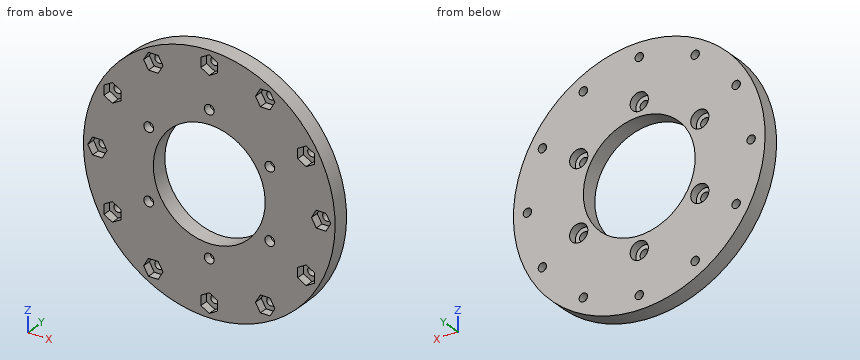
```python
from build123d import *

# Parameters (mm, degrees)
SKETCH1_R           = 45
BOSS_EXTRUDE1_DEPTH = 6
SKETCH3_R           = 1.75
CUT_EXTRUDE1_DEPTH  = 64.921827258
SKETCH4_R           = 3.25
CUT_EXTRUDE2_DEPTH  = 3
SKETCH5_R           = 1.5
CUT_EXTRUDE3_DEPTH  = 64.921827258
CUT_EXTRUDE4_DEPTH  = 3
SKETCH9_R           = 20
CUT_EXTRUDE5_DEPTH  = 64.921827258


with BuildPart() as part:
    # Sketch1 → Boss-Extrude1 (new body)
    with BuildSketch(Plane(origin=(0, 0, 0), x_dir=(1, 0, 0), z_dir=(0, 1, 0))):
        with Locations(Location((0, 0, 0), (0, 0, 270))):
            Circle(SKETCH1_R)
    extrude(amount=BOSS_EXTRUDE1_DEPTH)

    # Sketch3 → Cut-Extrude1 (cut, through all)
    with BuildSketch(Plane(origin=(0, 6, 0), x_dir=(1, 0, 0), z_dir=(0, 1, 0))):
        with Locations(Location((0, -25, 0), (0, 0, 270))):
            Circle(SKETCH3_R)
        with Locations(Location((-21.650635095, -12.5, 0), (0, 0, 270))):
            Circle(SKETCH3_R)
        with Locations(Location((-21.650635095, 12.5, 0), (0, 0, 270))):
            Circle(SKETCH3_R)
        with Locations(Location((0, 25, 0), (0, 0, 270))):
            Circle(SKETCH3_R)
        with Locations(Location((21.650635095, 12.5, 0), (0, 0, 270))):
            Circle(SKETCH3_R)
        with Locations(Location((21.650635095, -12.5, 0), (0, 0, 270))):
            Circle(SKETCH3_R)
    extrude(amount=-CUT_EXTRUDE1_DEPTH, mode=Mode.SUBTRACT)

    # Sketch4 → Cut-Extrude2 (cut)
    with BuildSketch(Plane(origin=(0, 6, 0), x_dir=(1, 0, 0), z_dir=(0, 1, 0))):
        with Locations(Location((0, -25, 0), (0, 0, 270))):
            Circle(SKETCH4_R)
        with Locations(Location((-21.650635095, -12.5, 0), (0, 0, 270))):
            Circle(SKETCH4_R)
        with Locations(Location((-21.650635095, 12.5, 0), (0, 0, 270))):
            Circle(SKETCH4_R)
        with Locations(Location((0, 25, 0), (0, 0, 270))):
            Circle(SKETCH4_R)
        with Locations(Location((21.650635095, 12.5, 0), (0, 0, 270))):
            Circle(SKETCH4_R)
        with Locations(Location((21.650635095, -12.5, 0), (0, 0, 270))):
            Circle(SKETCH4_R)
    extrude(amount=-CUT_EXTRUDE2_DEPTH, mode=Mode.SUBTRACT)

    # Sketch5 → Cut-Extrude3 (cut, through all)
    with BuildSketch(Plane(origin=(0, 6, 0), x_dir=(1, 0, 0), z_dir=(0, 1, 0))):
        with Locations(Location((0, -40, 0), (0, 0, 270))):
            Circle(SKETCH5_R)
        with Locations(Location((-20, -34.641016151, 0), (0, 0, 270))):
            Circle(SKETCH5_R)
        with Locations(Location((-34.641016151, -20, 0), (0, 0, 270))):
            Circle(SKETCH5_R)
        with Locations(Location((-40, 0, 0), (0, 0, 270))):
            Circle(SKETCH5_R)
        with Locations(Location((-34.641016151, 20, 0), (0, 0, 270))):
            Circle(SKETCH5_R)
        with Locations(Location((-20, 34.641016151, 0), (0, 0, 270))):
            Circle(SKETCH5_R)
        with Locations(Location((0, 40, 0), (0, 0, 270))):
            Circle(SKETCH5_R)
        with Locations(Location((20, 34.641016151, 0), (0, 0, 270))):
            Circle(SKETCH5_R)
        with Locations(Location((34.641016151, 20, 0), (0, 0, 270))):
            Circle(SKETCH5_R)
        with Locations(Location((40, 0, 0), (0, 0, 270))):
            Circle(SKETCH5_R)
        with Locations(Location((34.641016151, -20, 0), (0, 0, 270))):
            Circle(SKETCH5_R)
        with Locations(Location((20, -34.641016151, 0), (0, 0, 270))):
            Circle(SKETCH5_R)
    extrude(amount=-CUT_EXTRUDE3_DEPTH, mode=Mode.SUBTRACT)

    # Sketch6 → Cut-Extrude4 (cut)
    with BuildSketch(Plane.XZ):
        Polygon((-18.267949192, -37.641016151), (-16.535898385, -34.641016151), (-18.267949192, -31.641016151), (-21.732050808, -31.641016151), (-23.464101615, -34.641016151), (-21.732050808, -37.641016151), align=None)
        Polygon((0, -36.535898385), (-3, -38.267949192), (-3, -41.732050808), (0, -43.464101615), (3, -41.732050808), (3, -38.267949192), align=None)
        Polygon((-34.641016151, -23.464101615), (-31.641016151, -21.732050808), (-31.641016151, -18.267949192), (-34.641016151, -16.535898385), (-37.641016151, -18.267949192), (-37.641016151, -21.732050808), align=None)
        Polygon((-41.732050808, -3), (-38.267949192, -3), (-36.535898385, 0), (-38.267949192, 3), (-41.732050808, 3), (-43.464101615, 0), align=None)
        Polygon((-37.641016151, 18.267949192), (-34.641016151, 16.535898385), (-31.641016151, 18.267949192), (-31.641016151, 21.732050808), (-34.641016151, 23.464101615), (-37.641016151, 21.732050808), align=None)
        Polygon((-23.464101615, 34.641016151), (-21.732050808, 31.641016151), (-18.267949192, 31.641016151), (-16.535898385, 34.641016151), (-18.267949192, 37.641016151), (-21.732050808, 37.641016151), align=None)
        Polygon((-3, 41.732050808), (-3, 38.267949192), (0, 36.535898385), (3, 38.267949192), (3, 41.732050808), (0, 43.464101615), align=None)
        Polygon((18.267949192, 37.641016151), (16.535898385, 34.641016151), (18.267949192, 31.641016151), (21.732050808, 31.641016151), (23.464101615, 34.641016151), (21.732050808, 37.641016151), align=None)
        Polygon((34.641016151, 23.464101615), (31.641016151, 21.732050808), (31.641016151, 18.267949192), (34.641016151, 16.535898385), (37.641016151, 18.267949192), (37.641016151, 21.732050808), align=None)
        Polygon((41.732050808, 3), (38.267949192, 3), (36.535898385, 0), (38.267949192, -3), (41.732050808, -3), (43.464101615, 0), align=None)
        Polygon((37.641016151, -18.267949192), (34.641016151, -16.535898385), (31.641016151, -18.267949192), (31.641016151, -21.732050808), (34.641016151, -23.464101615), (37.641016151, -21.732050808), align=None)
        Polygon((23.464101615, -34.641016151), (21.732050808, -31.641016151), (18.267949192, -31.641016151), (16.535898385, -34.641016151), (18.267949192, -37.641016151), (21.732050808, -37.641016151), align=None)
    extrude(amount=-CUT_EXTRUDE4_DEPTH, mode=Mode.SUBTRACT)

    # Sketch9 → Cut-Extrude5 (cut, through all)
    with BuildSketch(Plane(origin=(0, 6, 0), x_dir=(1, 0, 0), z_dir=(0, 1, 0))):
        with Locations(Location((0, 0, 0), (0, 0, 270))):
            Circle(SKETCH9_R)
    extrude(amount=-CUT_EXTRUDE5_DEPTH, mode=Mode.SUBTRACT)


solid = part.part
```
The model under review builds one solid part; all positions refer to its coordinate system, in mm. Round coordinates to 2 decimals unless told otherwise and drop trailing zeros. Write each loop counter-clockwise with the first axis right and the second up, starting at its lowest first coordinate (ties: lowest second). Pieces come first, ordered by that corner, then holes.
(1) We need section A-A on z = 40. Give the boundary of the cut face in (x, y).
(2) We need section D-D on x = 9. Give the boundary of the cut face in (y, z), and give its area (3 significant figures).
(3) We need section B-B on x = -40. Give the boundary of the cut face in (y, z).
(4) Wall thickness on L1, parallel to X at y = 4.6, z = 0; L2, parallel to X at y = 1.85, z = -12.5; L3, parallel to Z at x = -36.5, y = 0.4: over which ranges is each line inside the solid? List them lowest first.
(5) Insertion check: pin 1 (1.5 mm diameter, centred on x = -20, y = 1.5, fed in from -Z); pin 2 (0.9 mm diameter, centred on y = 1, z = 20, fed in from -X); pin 3 (4.5 mm diameter, centred on x = 21.65, z = -12.5, fed in from +Y). Each pin has a flat end and moves straight along its axis. Give the tip position at first contact, or say it passes through.
(6) We need section C-C on z = 12.5. Give the boundary of the cut face in (x, y), and give its area (3 significant figures).
Findings below:
1. outline: (-20.62, 0) - (-3, 0) - (-3, 3) - (-1.5, 3) - (-1.5, 6) - (-20.62, 6) - close; (1.5, 3) - (3, 3) - (3, 0) - (20.62, 0) - (20.62, 6) - (1.5, 6) - close
2. outline: (0, -44.09) - (6, -44.09) - (6, -17.86) - (0, -17.86) - close; (0, 17.86) - (6, 17.86) - (6, 44.09) - (0, 44.09) - close
2. area: 315 mm2
3. outline: (0, -20.62) - (6, -20.62) - (6, -1.5) - (3, -1.5) - (3, -3) - (0, -3) - close; (0, 3) - (3, 3) - (3, 1.5) - (6, 1.5) - (6, 20.62) - (0, 20.62) - close
4. L1: x = -45 to -41.5, -38.5 to -20, 20 to 38.5, 41.5 to 45
4. L2: x = -43.23 to -23.4, -19.9 to -15.61, 15.61 to 19.9, 23.4 to 43.23
4. L3: z = -26.32 to -22.39, -17.61 to 17.61, 22.39 to 26.32
5. pin 1: stops at z = -40.67
5. pin 2: stops at x = -40.53
5. pin 3: stops at y = 3
6. outline: (-43.23, 0) - (-23.4, 0) - (-23.4, 3) - (-24.9, 3) - (-24.9, 6) - (-43.23, 6) - close; (-19.9, 0) - (-15.61, 0) - (-15.61, 6) - (-18.4, 6) - (-18.4, 3) - (-19.9, 3) - close; (15.61, 0) - (19.9, 0) - (19.9, 3) - (18.4, 3) - (18.4, 6) - (15.61, 6) - close; (23.4, 0) - (43.23, 0) - (43.23, 6) - (24.9, 6) - (24.9, 3) - (23.4, 3) - close
6. area: 271 mm2
